The model under review builds one solid part; all positions refer to its coordinate system, in mm. Face numbers are marked on the shaded views. A direction names the side the tool comes from. Coordinates: 2 decimals unless noted, no trailing zeros. Loops run counter-clockwise (first coordinate to the right, second up) from the corner with the lowest first, then second, coordinate; pieces in that order, holes last. Notation, with made-up numbers: (-30, 18.25) - (19, 18.25) arc R15 cw to (19, 24.25) - close; hole circle Ø2 at (-12, -40). An arc over 180 degrees is marked (long way). Answer in a Markdown table with one row per item. Add a question column.
(1) We need section B-B on z = -4. Write out the cut boundary in (x, y), plus the area to 3 significant figures.
(2) We need section D-D on x = -14. Write out the cut boundary in (y, z).
(3) We need section C-C on y = -3.75. Write out the cut boundary in (x, z).
(4) Machinability: for the marked faces 4 and 5, which of the approach directions +Z, -Z, +X, -X, +Y, -Y give a long, thin tool a straight path to every point of the face, cutting with its end or side? Answer none if there is none.
(5) For line 1 along Z through (x, y) = (0, -3.05); line 2 along Z through (x, y) = (-1.5, -2); line 3 along Y through (x, z) = (1, -12.5), list the stretches that pass through material, from the lowest coordinate up.
(6) Mouldability with a two-part tool opening along X and no side actions: class the marked faces 1, 2 and 3 as +X half, -X half, draft (parallel to the pull), parting line (faces both ways), or undercut.
(7) We need section A-A on x = 0. Write out the cut boundary in (y, z), plus the area to 3 significant figures.
(8) For P1, Ø2, axis at y = -5, z = -8, coming from the +X side; P2, Ø2, axis at y = -3, z = -18.5, coming from the -X side; P3, Ø1, axis at x = 15, z = -6.5, coming from the +Y side; P4, Ø3, axis at x = 4, y = -3, coming from the -Z side, all flat-tipped, find the tip position at first contact; note any pin that passes through.
from build123d import *

# Parameters (mm, degrees)
F0_R     = 26
F1_DEPTH = 5
F2_R     = 12.5
F3_DEPTH = 7
F4_R     = 3
F5_DEPTH = 25
F6_R     = 8
F7_DEPTH = 25


with BuildPart() as f1:
    # F0 (on Front) → F1 (new body)
    with BuildSketch(Plane.XZ):
        Circle(F0_R)
    extrude(amount=F1_DEPTH)

    # F2 (on face) → F3 (join)
    with BuildSketch(Plane.XZ.offset(5)):
        Circle(F2_R)
    extrude(amount=F3_DEPTH)

    # F4 (on face) → F5 (cut)
    with BuildSketch(Plane.XZ.offset(5)):
        with Locations((0, 17.5)):
            Circle(F4_R)
        with Locations((-15.155445, -8.75)):
            Circle(F4_R)
        with Locations((15.155445, -8.75)):
            Circle(F4_R)
    extrude(amount=-F5_DEPTH, mode=Mode.SUBTRACT)

    # F6 (on face) → F7 (cut)
    with BuildSketch(Plane.XZ.offset(12)):
        Circle(F6_R)
    extrude(amount=-F7_DEPTH, mode=Mode.SUBTRACT)


solid = f1.part
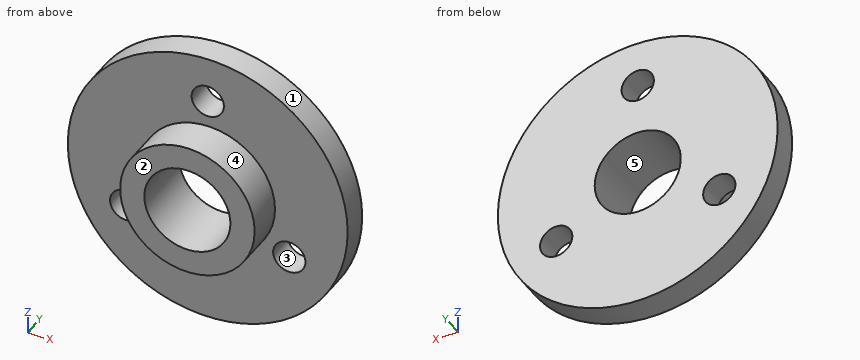
Outcome:
| question | item | result |
|---|---|---|
| 1 | outline | (-25.69, -5) - (-11.84, -5) - (-11.84, -12) - (-6.93, -12) - (-6.93, 0) - (-25.69, 0) - close; (6.93, -12) - (11.84, -12) - (11.84, -5) - (25.69, -5) - (25.69, 0) - (6.93, 0) - close |
| 1 | area | 256 mm² |
| 2 | outline | (-5, -21.91) - (0, -21.91) - (0, -11.52) - (-5, -11.52) - close; (-5, -5.98) - (0, -5.98) - (0, 21.91) - (-5, 21.91) - close |
| 3 | outline | circle Ø52 at (0, 0); hole circle Ø6 at (-15.16, -8.75); hole circle Ø16 at (0, 0); hole circle Ø6 at (0, 17.5); hole circle Ø6 at (15.16, -8.75) |
| 4 | face 4 | -Y |
| 4 | face 5 | +Y, -Y |
| 5 | line 1 | -26 to -8, 8 to 14.5, 20.5 to 26 |
| 5 | line 2 | -25.96 to -7.86, 7.86 to 14.9, 20.1 to 25.96 |
| 5 | line 3 | -5 to 0 |
| 6 | face 1 | parting line |
| 6 | face 2 | draft |
| 6 | face 3 | undercut |
| 7 | outline | (-12, -12.5) - (-5, -12.5) - (-5, -26) - (0, -26) - (0, -8) - (-12, -8) - close; (-12, 8) - (0, 8) - (0, 14.5) - (-5, 14.5) - (-5, 12.5) - (-12, 12.5) - close; (-5, 20.5) - (0, 20.5) - (0, 26) - (-5, 26) - close |
| 7 | area | 213 mm² |
| 8 | P1 | x = 25.04 |
| 8 | P2 | x = -19.23 |
| 8 | P3 | through |
| 8 | P4 | z = -25.88 |
